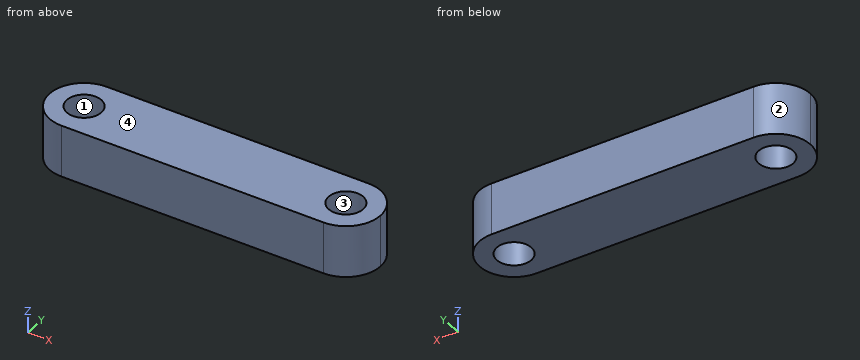
from build123d import *

# Parameters (mm, degrees)
IZIM1_W                     = 192
IZIM1_H                     = 40
IZIM1_R                     = 10
Y_KSEKLIK_EKSTR_ZYON1_DEPTH = 15
RADYUS1_R                   = 20


with BuildPart() as part:
    # Çizim1 → Yükseklik-Ekstrüzyon1 (new, symmetric)
    with BuildSketch(Plane.XY):
        Rectangle(IZIM1_W, IZIM1_H)
        with Locations((-76, 0)):
            Circle(IZIM1_R, mode=Mode.SUBTRACT)
        with Locations(Location((76, 0, 0), (0, 0, 180))):
            Circle(IZIM1_R, mode=Mode.SUBTRACT)
    extrude(amount=Y_KSEKLIK_EKSTR_ZYON1_DEPTH, both=True)

    # Radyus1
    radyus1_edges = [part.edges().sort_by_distance(p)[0] for p in [
        (-96, -20, 0),
        (-96, 20, 0),
        (96, -20, 0),
        (96, 20, 0),
    ]]
    fillet(radyus1_edges, radius=RADYUS1_R - 0.0001)  # a hair under: the kernel refuses the full size


solid = part.part
For this review, take the finished solid that the model builds, in its own axes (mm). Face numbers are marked on the shaded views. Coordinates: 2 decimals unless noted, no trailing zeros. Loops run counter-clockwise (first coordinate to the right, second up) from the corner with the lowest first, then second, coordinate; pieces in that order, holes last. Notation, with made-up numbers: (-22, 78) - (-14, 78) arc R22 cw to (-14, 91) - close; hole circle Ø10 at (61.5, 61.5). An arc over 180 degrees is marked (long way). Use a Markdown table: item, result. Add a question column.
Item 1: Mouldability with a two-part tool opening along X and no side actions: class the marked faces 1, 2, 3 and 4 as pulls with the +X half, pulls with the -X half, needs draft (parallel to the pull), parting line crosses it, or undercut.
Item 2: We need section A-A (y = 4). Give the boundary of the cut face in (x, z), and give its area (3 significant figures).
Item 3: We need section B-B (x = -74). Give the boundary of the cut face in (y, z).
Item 4: For line 1 (X direction, y = 8, z = 8.25); line 2 (X direction, y = 0.5, z = -8.75); line 3 (Y direction, x = -76, z = -3.5), list the stretches that pass through material, from the lowest coordinate up.
Item 5: We need section D-D (y = -16). Give the boundary of the cut face in (x, z).
Item 6: Insertion check: pin 1 Ø5 at (y, z) = (-13, 12) entering from +X; pin 2 Ø23 at (x, y) = (76, 0) entering from -Z; pin 3 Ø1 at (y, z) = (3, 2.5) entering from -X. Each pin has a flat end and moves straight along its axis. Give the tip position at first contact, or say it passes through.
Item 7: We need section C-C (z = -2). Give the number of separate pieces and of enclosed holes in the cut face, and give its area (3 significant figures).
Results list:
| question | item | result |
|---|---|---|
| 1 | face 1 | undercut |
| 1 | face 2 | pulls with the -X half |
| 1 | face 3 | undercut |
| 1 | face 4 | needs draft |
| 2 | outline | (-95.6, -15) - (-85.17, -15) - (-85.17, 15) - (-95.6, 15) - close; (-66.83, -15) - (66.83, -15) - (66.83, 15) - (-66.83, 15) - close; (85.17, -15) - (95.6, -15) - (95.6, 15) - (85.17, 15) - close |
| 2 | area | 4,640 mm^2 |
| 3 | outline | (-20, -15) - (-9.8, -15) - (-9.8, 15) - (-20, 15) - close; (9.8, -15) - (20, -15) - (20, 15) - (9.8, 15) - close |
| 4 | line 1 | x = -94.33 to -82, -70 to 70, 82 to 94.33 |
| 4 | line 2 | x = -95.99 to -85.99, -66.01 to 66.01, 85.99 to 95.99 |
| 4 | line 3 | y = -20 to -10, 10 to 20 |
| 5 | outline | (-88, -15) - (88, -15) - (88, 15) - (-88, 15) - close |
| 6 | pin 1 | stops at x = 93.02 |
| 6 | pin 2 | stops at z = -15 |
| 6 | pin 3 | stops at x = -95.84 |
| 7 | separate pieces | 1 |
| 7 | enclosed holes | 2 |
| 7 | area | 6,710 mm^2 |
